Here's the drawing with two shaded views (mm, measured from the low corner). I have some questions. A direction names the side the tool comes from. Round coordinates to 2 decimals unless told otherwise and drop trailing zeros. Loops run counter-clockwise (first coordinate to the right, second up) from the corner with the lowest first, then second, coordinate; pieces in that order, holes last. Notation, with made-up numbers: M 84.5,78 L 119.5,78 A16 ccw 119.5,92 Z; hole C -6,8 d9. An arc over 180 degrees is marked long. One line per item, written item: value. Start each with the question number.
Q1. Imagine slicing it at C-C (z = 71.5). Please give me the cut outline in (x, y), then the cut area to 3 significant figures.
Q2. Which directions (+Z, -Z, +X, -X, +Y, -Y) give clear straight access to the entire face, cutting with the end or side of a thin tool? Please do the marked faces 1 and 2.
Q3. Imagine slicing it at A-A (y = 38.1). Please give me the cut outline in (x, z).
Q4. Thinking about a two-plate mould opening in Y: for the marked faces 3, 4 and 5, which applies, released by +Y, released by -Y, zero draft, split by the parting line, or undercut?
Q5. Please list where this line runs through material, in increasing order: line 1 along Z through (x, y) = (38, 73).
Q6. Imagine slicing it at D-D (z = 36.5). Please give me the cut outline in (x, y).
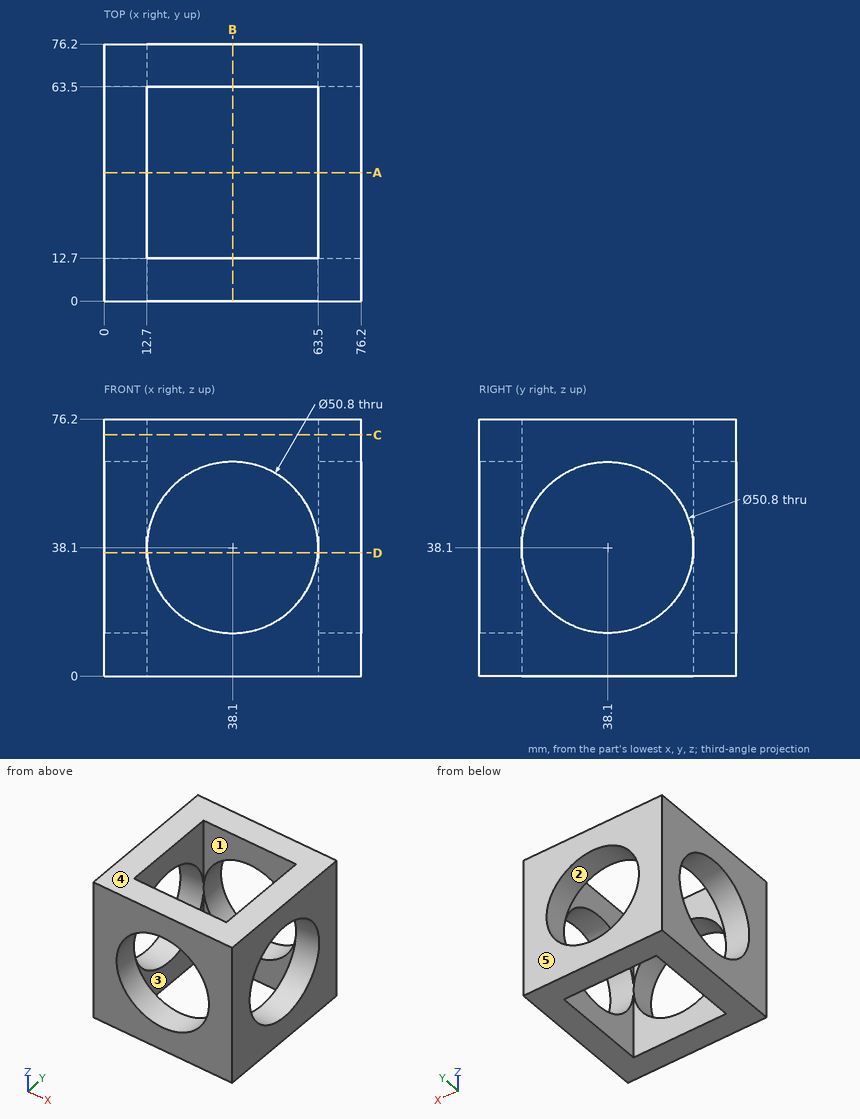
Report:
1. outline: M 0,0 L 76.2,0 L 76.2,76.2 L 0,76.2 Z; hole M 12.7,12.7 L 63.5,12.7 L 63.5,63.5 L 12.7,63.5 Z
1. area: 3,230 mm²
2. face 1: +Z, -Z
2. face 2: +Y, -Y
3. outline: M 0,0 L 12.7,0 L 12.7,12.7 L 0,12.7 Z; M 0,63.5 L 12.7,63.5 L 12.7,76.2 L 0,76.2 Z; M 63.5,0 L 76.2,0 L 76.2,12.7 L 63.5,12.7 Z; M 63.5,63.5 L 76.2,63.5 L 76.2,76.2 L 63.5,76.2 Z
4. face 3: undercut
4. face 4: zero draft
4. face 5: released by +Y
5. line 1: z = 0 to 12.7, 63.5 to 76.2
6. outline: M 0,0 L 12.75,0 L 12.75,12.7 L 12.7,12.7 L 12.7,12.75 L 0,12.75 Z; M 0,63.45 L 12.7,63.45 L 12.7,63.5 L 12.75,63.5 L 12.75,76.2 L 0,76.2 Z; M 63.45,0 L 76.2,0 L 76.2,12.75 L 63.5,12.75 L 63.5,12.7 L 63.45,12.7 Z; M 63.45,63.5 L 63.5,63.5 L 63.5,63.45 L 76.2,63.45 L 76.2,76.2 L 63.45,76.2 Z
